Read the model definition and answer for the solid it produces. Units are mm, in the model's axes. Face numbers are marked on the shaded views. A direction names the side the tool comes from. Coordinates: 2 decimals unless noted, no trailing zeros. Write each loop counter-clockwise with the first axis right and the second up, starting at its lowest first coordinate (ties: lowest second). Pieces come first, ordered by that corner, then holes. Notation, with made-up numbers: (-39.75, 15) -> (2.25, 15) arc R14 ccw to (2.25, 38) -> close; hole circle Ø1 at (-25.75, 44.5). An arc over 180 degrees is marked (long way). Answer as a JSON object with one key per item and string values. Group by question number.
(1) Find section B-B (x = -1.5). Give the vertices of the cut face in (y, z) (3 decimals).
(2) Find section C-C (z = 20.76). Give the vertices of the cut face in (x, y), then the cut area to 3 significant figures.
(3) Find section D-D (x = 3.5). Give the vertices of the cut face in (y, z), then the cut area to 3 significant figures.
(4) Flat-ended cylindrical pins translate along their axes: P1, Ø1.5, axis at y = -1.5, z = 27.5, coming from the -X side; P2, Ø5.5, axis at x = -2, z = 20.5, coming from the +Y side; P3, Ø3.5, axis at y = 0, z = 22, coming from the -X side. Find the tip coordinate at first contact, or state that the pin passes through.
(5) Find section A-A (y = 1.5). Give the vertices of the cut face in (x, z).
(6) Which of the six approach directions +Z, -Z, +X, -X, +Y, -Y give full straight-line access (tool end or side, diameter ignored) to the marked faces 1 and 2?
(7) Straight lines are drawn through the part: L1, parallel to Z at x = -1.5, y = -3.45 (3 decimals); L2, parallel to Y at x = 2.6, z = 10.76; L3, parallel to Y at x = 0.5, z = 5.5. For each, find the intervals that lie inside material, in ascending order.
(8) For a pull along X with two mould halves and no side action, classify the marked faces 3, 4, 5 and 6 as +X half, -X half, draft (parallel to the pull), parting line (faces both ways), or undercut.
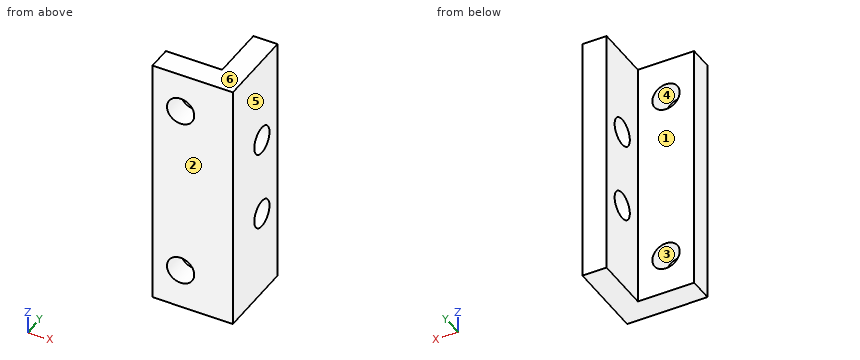
from build123d import *

# Parameters (mm, degrees)
EXTRUDE_1_DEPTH    = 31.52
HOLE_WIZARD_M3_1_D = 3.4
HOLE_WIZARD_M3_2_D = 3.4


with BuildPart() as part:
    # ｽｹｯﾁ1 → ﾎﾞｽ - 押し出し1 (new body)
    with BuildSketch(Plane.XY):
        Polygon((-5, -2), (2, -2), (2, 5), (5, 5), (5, -5), (-5, -5), align=None)
    extrude(amount=EXTRUDE_1_DEPTH)

    # M3 すきま穴1 (through all)
    with Locations(Plane(origin=(0, -2, 0), x_dir=(1, 0, 0), z_dir=(0, 1, 0))):
        with Locations((-1.5, -4.935), (-1.5, -26.585)):
            Hole(HOLE_WIZARD_M3_1_D / 2)

    # M3 すきま穴2 (through all)
    with Locations(Plane.ZY.offset(-2)):
        with Locations((10.76, 1.5), (20.76, 1.5)):
            Hole(HOLE_WIZARD_M3_2_D / 2)


solid = part.part
Results below:
{
 "1": {"outline": "(-5, 0) -> (-2, 0) -> (-2, 3.235) -> (-5, 3.235) -> close; (-5, 6.635) -> (-2, 6.635) -> (-2, 24.885) -> (-5, 24.885) -> close; (-5, 28.285) -> (-2, 28.285) -> (-2, 31.52) -> (-5, 31.52) -> close"},
 "2": {"outline": "(-5, -5) -> (5, -5) -> (5, -0.2) -> (2, -0.2) -> (2, -2) -> (-5, -2) -> close; (2, 3.2) -> (5, 3.2) -> (5, 5) -> (2, 5) -> close", "area": "40.8 mm2"},
 "3": {"outline": "(-5, 0) -> (5, 0) -> (5, 31.52) -> (-5, 31.52) -> close; hole circle Ø3.4 at (1.5, 10.76); hole circle Ø3.4 at (1.5, 20.76)", "area": "297 mm2"},
 "4": {"P1": "stops at x = -5", "P2": "stops at y = -2", "P3": "stops at x = 2"},
 "5": {"outline": "(2, 0) -> (5, 0) -> (5, 9.06) -> (2, 9.06) -> close; (2, 12.46) -> (5, 12.46) -> (5, 19.06) -> (2, 19.06) -> close; (2, 22.46) -> (5, 22.46) -> (5, 31.52) -> (2, 31.52) -> close"},
 "6": {"face 1": "+Z, -Z, -X, +Y", "face 2": "+Z, -Z, +X, -X, -Y"},
 "7": {"L1": "z = 0 to 3.235, 6.635 to 24.885, 28.285 to 31.52", "L2": "y = -5 to -0.2, 3.2 to 5", "L3": "y = -5 to -2"},
 "8": {"face 3": "undercut", "face 4": "undercut", "face 5": "+X half", "face 6": "draft"}
}
